Verification items for the finished model (mm, model axes). Give positions to 0.01 mm unless a question says otherwise; leave off trailing zeros. Write each loop counter-clockwise with the first axis right and the second up, starting at its lowest first coordinate (ties: lowest second). Pieces come first, ordered by that corner, then holes.
from build123d import *

# Parameters (mm, degrees)
SKETCH1_W          = 315.9125
SKETCH1_H          = 265.1125
SKETCH1_R          = 3.3782
SKETCH1_R_2        = 14.351
SKETCH1_R_3        = 6.35
SKETCH1_R_4        = 2.4892
BASE_FLANGE1_DEPTH = 3.175
SKETCH2_W          = 29.4
SKETCH2_H          = 265.1125
CUT_EXTRUDE1_DEPTH = 413.426267274


# Sheet-metal steps are written as plain solids
with BuildPart() as part:
    # Sketch1 → Base-Flange1 (new body)
    with BuildSketch(Plane(origin=(0, 0, 0), x_dir=(1, 0, 0), z_dir=(0, 1, 0))):
        with Locations((-157.95625, 132.55625)):
            Rectangle(SKETCH1_W, SKETCH1_H)
        with Locations(Location((-254, 64.29375, 0), (0, 0, 270))):
            Circle(SKETCH1_R, mode=Mode.SUBTRACT)
        with Locations(Location((-254, 89.69375, 0), (0, 0, 270))):
            Circle(SKETCH1_R, mode=Mode.SUBTRACT)
        with Locations(Location((-254, 153.19375, 0), (0, 0, 270))):
            Circle(SKETCH1_R, mode=Mode.SUBTRACT)
        with Locations(Location((-254, 178.59375, 0), (0, 0, 270))):
            Circle(SKETCH1_R, mode=Mode.SUBTRACT)
        with Locations(Location((-61.9125, 64.29375, 0), (0, 0, 90))):
            Circle(SKETCH1_R, mode=Mode.SUBTRACT)
        with Locations(Location((-61.9125, 89.69375, 0), (0, 0, 90))):
            Circle(SKETCH1_R, mode=Mode.SUBTRACT)
        with Locations(Location((-61.9125, 153.19375, 0), (0, 0, 90))):
            Circle(SKETCH1_R, mode=Mode.SUBTRACT)
        with Locations(Location((-61.9125, 178.59375, 0), (0, 0, 90))):
            Circle(SKETCH1_R, mode=Mode.SUBTRACT)
        with Locations(Location((-157.95625, 145.25625, 0), (0, 0, 270))):
            Circle(SKETCH1_R_2, mode=Mode.SUBTRACT)
        with Locations(Location((-157.95625, 84.29625, 0), (0, 0, 270))):
            Circle(SKETCH1_R_3, mode=Mode.SUBTRACT)
        with Locations(Location((-176.37125, 114.26825, 0), (0, 0, 270))):
            Circle(SKETCH1_R_4, mode=Mode.SUBTRACT)
        with Locations(Location((-115.91925, 114.26825, 0), (0, 0, 270))):
            Circle(SKETCH1_R_4, mode=Mode.SUBTRACT)
        with Locations(Location((-115.91925, 50.76825, 0), (0, 0, 270))):
            Circle(SKETCH1_R_4, mode=Mode.SUBTRACT)
        with Locations(Location((-176.37125, 50.76825, 0), (0, 0, 270))):
            Circle(SKETCH1_R_4, mode=Mode.SUBTRACT)
        with Locations(Location((-234.15625, 7.9375, 0), (0, 0, 270))):
            Circle(SKETCH1_R, mode=Mode.SUBTRACT)
        with Locations(Location((-157.95625, 7.9375, 0), (0, 0, 270))):
            Circle(SKETCH1_R, mode=Mode.SUBTRACT)
        with Locations(Location((-81.75625, 7.9375, 0), (0, 0, 270))):
            Circle(SKETCH1_R, mode=Mode.SUBTRACT)
        with Locations(Location((-157.95625, 257.175, 0), (0, 0, 270))):
            Circle(SKETCH1_R, mode=Mode.SUBTRACT)
        with Locations(Location((-81.75625, 257.175, 0), (0, 0, 270))):
            Circle(SKETCH1_R, mode=Mode.SUBTRACT)
        with Locations(Location((-234.15625, 257.175, 0), (0, 0, 270))):
            Circle(SKETCH1_R, mode=Mode.SUBTRACT)
        with Locations(Location((-227.80625, 84.29625, 0), (0, 0, 270))):
            Circle(SKETCH1_R, mode=Mode.SUBTRACT)
        with Locations(Location((-88.10625, 84.29625, 0), (0, 0, 270))):
            Circle(SKETCH1_R, mode=Mode.SUBTRACT)
        with Locations(Location((-273.84375, 223.8375, 0), (0, 0, 270))):
            Circle(SKETCH1_R, mode=Mode.SUBTRACT)
        with Locations(Location((-273.84375, 135.73125, 0), (0, 0, 270))):
            Circle(SKETCH1_R, mode=Mode.SUBTRACT)
        with Locations(Location((-273.84375, 47.625, 0), (0, 0, 270))):
            Circle(SKETCH1_R, mode=Mode.SUBTRACT)
        with Locations(Location((-42.06875, 223.8375, 0), (0, 0, 90))):
            Circle(SKETCH1_R, mode=Mode.SUBTRACT)
        with Locations(Location((-42.06875, 135.73125, 0), (0, 0, 90))):
            Circle(SKETCH1_R, mode=Mode.SUBTRACT)
        with Locations(Location((-42.06875, 47.625, 0), (0, 0, 90))):
            Circle(SKETCH1_R, mode=Mode.SUBTRACT)
    extrude(amount=-BASE_FLANGE1_DEPTH)

    # Sketch2 → Cut-Extrude1 (cut, through all)
    with BuildSketch(Plane(origin=(0, 0, 0), x_dir=(1, 0, 0), z_dir=(0, 1, 0))):
        with Locations((-301.2125, 132.55625)):
            Rectangle(SKETCH2_W, SKETCH2_H)
        with Locations((-14.7, 132.55625)):
            Rectangle(SKETCH2_W, SKETCH2_H)
    extrude(amount=-CUT_EXTRUDE1_DEPTH, mode=Mode.SUBTRACT)


solid = part.part
Item 1: Release check for a two-part mould opening along Z. For faces 1 (the face through (-87.96, -1.57, -87.67)), 2 (the face through (-131, -3.175, -134)) record: released by +Z, released by -Z, zero draft, split by the parting line, or undercut.
Answer key:
face 1: undercut
face 2: zero draft
Item 2: Scan lines: line 1 along Z through (x, y) = (-228, -1.7); line 2 along X through (y, z) = (-2.75, -177); line 3 along Z through (x, y) = (-233, -0.85). Record each from-to range of solid material in increasing order.
Answer key:
line 1: z = -265.11 to -87.67, -80.92 to 0
line 2: x = -286.51 to -256.98, -251.02 to -64.89, -58.93 to -29.4
line 3: z = -265.11 to -260.35, -254 to -11.11, -4.76 to 0
Item 3: Sectioned sample at A-A on x = -254. Record the cut outline in (y, z) (1 decimal), then the cut area to 3 significant figures.
Answer key:
outline: (-3.2, -265.1) - (0, -265.1) - (0, -182) - (-3.2, -182) - close; (-3.2, -175.2) - (0, -175.2) - (0, -156.6) - (-3.2, -156.6) - close; (-3.2, -149.8) - (0, -149.8) - (0, -93.1) - (-3.2, -93.1) - close; (-3.2, -86.3) - (0, -86.3) - (0, -67.7) - (-3.2, -67.7) - close; (-3.2, -60.9) - (0, -60.9) - (0, 0) - (-3.2, 0) - close
area: 756 mm2
Item 4: Sectioned sample at B-B on y = -2.1. State how many separate pieces and enclosed holes the cut face has, then the cut area to 3 significant figures.
Answer key:
separate pieces: 1
enclosed holes: 28
area: 66,500 mm2
